Can you work these out from the model? Positions are in its coordinate system, mm. Face numbers are marked on the shaded views. Give positions to 0.01 mm unless a question says otherwise; leave off trailing zeros. Order: outer loops, then holes, each group sorted by start corner. A loop starts at its lowest first (then second) coordinate and runs counter-clockwise, first axis right, second up. Notation, with made-up numbers: (-26.75, 88.25) - (-22.75, 88.25) arc R16 ccw to (-22.75, 93.25) - close; hole circle Ø3 at (13, 79). An arc over 180 degrees is marked (long way). Return JSON: item names as keys, results as strings.
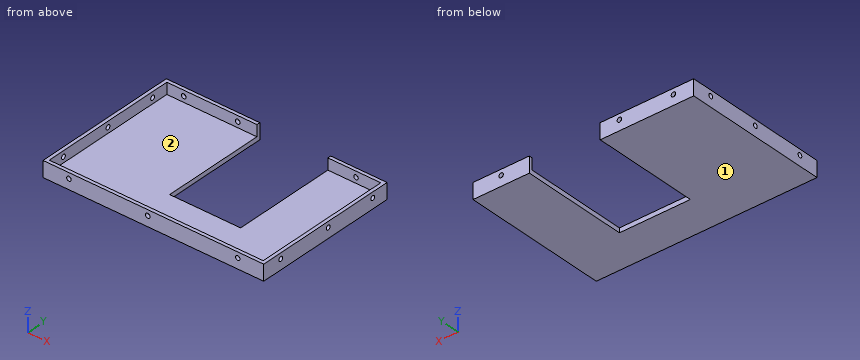
```python
from build123d import *

# Parameters (mm, degrees)
F1_DEPTH  = 4
F3_DEPTH  = 10
F4_R      = 2
F5_DEPTH  = 5
F7_R      = 2
F8_DEPTH  = 5
F6_R      = 2
F9_DEPTH  = 5
F10_R     = 2
F11_DEPTH = 5


with BuildPart() as f1:
    # F0 (on Top) → F1 (new body)
    with BuildSketch(Plane.XY):
        Polygon((-14.729894, 40.995409), (-97.729894, 40.995409), (-97.729894, -89.004591), (98.270106, -89.004591), (98.270106, 40.995409), (48.270106, 40.995409), (48.270106, -54.004591), (-14.729894, -54.004591), align=None)
    extrude(amount=F1_DEPTH)

    # F2 (on face) → F3 (join)
    with BuildSketch(Plane.XY.offset(4)):
        Polygon((-94.729894, -86.004591), (-94.729894, 37.995409), (-14.729894, 37.995409), (-14.729894, 40.995409), (-97.729894, 40.995409), (-97.729894, -89.004591), (98.270106, -89.004591), (98.270106, 40.995409), (48.270106, 40.995409), (48.270106, 37.995409), (95.270106, 37.995409), (95.270106, -86.004591), align=None)
    extrude(amount=F3_DEPTH)

    # F4 (on face) → F5 (cut)
    with BuildSketch(Plane.YZ.offset(-94.729894)):
        with Locations((22.995409, 9)):
            Circle(F4_R)
        with Locations((-24.004591, 9)):
            Circle(F4_R)
        with Locations((-71.004591, 9)):
            Circle(F4_R)
    extrude(amount=-F5_DEPTH, mode=Mode.SUBTRACT)

    # F7 (on face) → F8 (cut)
    with BuildSketch(Plane(origin=(95.270106, 0, 0), x_dir=(0, -1, 0), z_dir=(-1, 0, 0))):
        with Locations((71.004591, 9)):
            Circle(F7_R)
        with Locations((21.004591, 9)):
            Circle(F7_R)
        with Locations((-25.995409, 9)):
            Circle(F7_R)
    extrude(amount=-F8_DEPTH, mode=Mode.SUBTRACT)

    # F6 (on face) → F9 (cut)
    with BuildSketch(Plane.XZ.offset(-37.995409)):
        with Locations((-79.729894, 9)):
            Circle(F6_R)
        with Locations((-31.729894, 9)):
            Circle(F6_R)
        with Locations((73.270106, 9)):
            Circle(F6_R)
    extrude(amount=-F9_DEPTH, mode=Mode.SUBTRACT)

    # F10 (on face) → F11 (cut)
    with BuildSketch(Plane(origin=(0, -86.004591, 0), x_dir=(-1, 0, 0), z_dir=(0, 1, 0))):
        with Locations((-75.270106, 9)):
            Circle(F10_R)
        with Locations((4.729894, 9)):
            Circle(F10_R)
        with Locations((74.729894, 9)):
            Circle(F10_R)
    extrude(amount=-F11_DEPTH, mode=Mode.SUBTRACT)


solid = f1.part
```
1. If I drill on L1, parallel to X at y = -15, z = 4.5; L2, parallel to Y at x = 64, z = 6.25; L3, parallel to Z at x = -21, y = -83, over which ranges is the centre line in solid material (lowest first)? Write a range as [from, to].
Checks:
{"L1": "[-97.73, -94.73], [95.27, 98.27]", "L2": "[-89, -86], [38, 41]", "L3": "[0, 4]"}
2. Thinking about a two-plate mould opening in Y: for the marked faces 1 and 2, which applies, +Y half, -Y half, draft (parallel to the pull), parting line (faces both ways), or undercut?
Checks:
{"face 1": "draft", "face 2": "undercut"}
3. Suppose I cut it at A-A (y = -58). List the corners of the cut face in (x, z) for me.
Checks:
{"outline": "(-97.73, 0) - (98.27, 0) - (98.27, 14) - (95.27, 14) - (95.27, 4) - (-94.73, 4) - (-94.73, 14) - (-97.73, 14) - close"}
4. Suppose I cut it at B-B (x = 30). List the corners of the cut face in (y, z) for me.
Checks:
{"outline": "(-89, 0) - (-54, 0) - (-54, 4) - (-86, 4) - (-86, 14) - (-89, 14) - close"}
5. Suppose I cut it at D-D (x = -58). List the corners of the cut face in (y, z) for me, plus the area to 3 significant figures.
Checks:
{"outline": "(-89, 0) - (41, 0) - (41, 14) - (38, 14) - (38, 4) - (-86, 4) - (-86, 14) - (-89, 14) - close", "area": "580 mm^2"}
6. For pin 1 Ø3 at (x, z) = (-4.73, 9) entering from -Y; pin 2 Ø2.5 at (y, z) = (26, 9) entering from +X; pin 3 Ø3.5 at (x, z) = (-31.73, 9) entering from +Y, each with a flat end and sliding along its axis, tell me the tip position at first contact or that it passes through.
Checks:
{"pin 1": "through", "pin 2": "x = -94.73", "pin 3": "y = -86"}
7. Suppose I cut it at C-C (z = 9). State how many separate pieces and enclosed holes the cut face has, plus the area to 3 significant figures.
Checks:
{"separate pieces": "13", "enclosed holes": "0", "area": "1,590 mm^2"}
